Here's the drawing with two shaded views (mm, measured from the low corner). I have some questions. A direction names the side the tool comes from. Coordinates: 2 decimals unless noted, no trailing zeros. Write each loop counter-clockwise with the first axis right and the second up, starting at its lowest first coordinate (ties: lowest second). Pieces come first, ordered by that corner, then holes. Notation, with made-up numbers: (1, 42.5) -> (60, 42.5) arc R28 ccw to (60, 66.5) -> close; hole circle Ø2 at (10.25, 37). An arc over 180 degrees is marked (long way). Use one line per item in the form item = value.
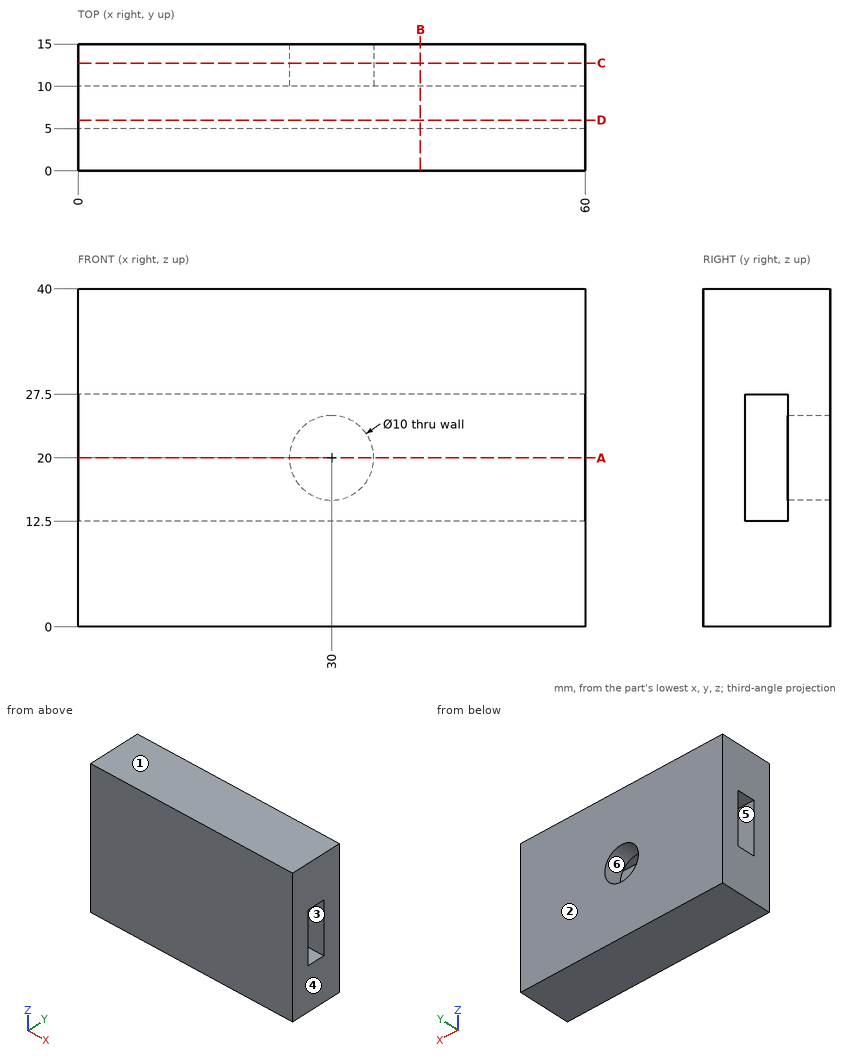
Q1. Suppose I cut it at C-C (y = 12.75). Write out the boundary of the cut face in (x, z), then the cut area to 3 significant figures.
Return value:
outline = (0, 0) -> (60, 0) -> (60, 40) -> (0, 40) -> close; hole circle Ø10 at (30, 20)
area = 2,320 mm2
Q2. For the marked faces 4, 5 and 6, which set-ups out of +Z, -Z, +X, -X, +Y, -Y let a thin tool reach every point of the face, with its end or its side?
Return value:
face_4 = +Z, -Z, +X, +Y, -Y
face_5 = +X, -X
face_6 = +Y
Q3. Thinking about a two-plate mould opening in Z: for the marked faces 1, 2 and 3, which applies, released by +Z, released by -Z, zero draft, split by the parting line, or undercut?
Return value:
face_1 = released by +Z
face_2 = zero draft
face_3 = undercut
Q4. If I drill on line 1 (Z direction, x = 7, y = 8.25); line 2 (X direction, y = 12.5, z = 20); line 3 (Y direction, x = 21, z = 26), over which ranges is the centre line in solid material (lowest first)? Write a range as from..to.
Return value:
line_1 = 0..12.5, 27.5..40
line_2 = 0..25, 35..60
line_3 = 0..5, 10..15
Q5. Suppose I cut it at A-A (z = 20). Write out the boundary of the cut face in (x, y).
Return value:
outline = (0, 0) -> (60, 0) -> (60, 5) -> (0, 5) -> close; (0, 10) -> (25, 10) -> (25, 15) -> (0, 15) -> close; (35, 10) -> (60, 10) -> (60, 15) -> (35, 15) -> close
Q6. Suppose I cut it at D-D (y = 6). Write out the boundary of the cut face in (x, z).
Return value:
outline = (0, 0) -> (60, 0) -> (60, 12.5) -> (0, 12.5) -> close; (0, 27.5) -> (60, 27.5) -> (60, 40) -> (0, 40) -> close
Q7. Will this pin go through, and if not, where does the flat tip stop? pin 1 (3 mm diameter, centred on x = 16, y = 5.5, fed in from -Z).
Return value:
pin_1 = 0
Q8. Suppose I cut it at B-B (x = 40.5). Write out the boundary of the cut face in (y, z).
Return value:
outline = (0, 0) -> (15, 0) -> (15, 40) -> (0, 40) -> close; hole (5, 12.5) -> (10, 12.5) -> (10, 27.5) -> (5, 27.5) -> close
